Could you check a few things on this model? Use its own coordinates, in mm. A direction names the side the tool comes from. Round coordinates to 2 decimals unless told otherwise and drop trailing zeros. Loops run counter-clockwise (first coordinate to the right, second up) from the corner with the lowest first, then second, coordinate; pieces in that order, holes last. Notation, with made-up numbers: M 16,11.25 L 62,11.25 A13 cw 62,27.25 Z; hole C 72,-19 d6. An arc over 180 degrees is marked long. One line per item, written item: value. Start each with the question number.
Q1. Imagine slicing it at C-C (y = -18.95). Please give me the cut outline in (x, z).
Q2. Thinking about a two-plate mould opening in Y: for faces 1 (the face through (1.52, -22.24, 19.24)), 2 (the face through (1, -25, 28)), 3 (the face through (1, -35, 23)), which applies, released by +Y, released by -Y, zero draft, split by the parting line, or undercut?
Q3. I'm going to push flat-ended pins straight in: pin 1 Ø1.4 at (x, y) = (1, -33) entering from +Z; pin 2 Ø3 at (y, z) = (0, -21) entering from +X; pin 3 Ø1.5 at (x, z) = (1.5, 26.5) entering from +Y; pin 4 Ø0.9 at (x, y) = (1.5, -17) entering from -Z. Where does each tip first touch, or does it pass through?
Q4. Please list where these lines run through material, in increasing order: line 1 along Y through (x, z) = (0.65, -4); line 2 along Y through (x, z) = (0.4, 25.5); line 3 along Y through (x, z) = (0.95, 21).
Q5. Imagine slicing it at B-B (y = 0). Please give me the cut outline in (x, z).
Q6. Imagine slicing it at A-A (z = -21). Please give me the cut outline in (x, y).
Q7. Which directions (+Z, -Z, +X, -X, +Y, -Y) give clear straight access to the entire face, cutting with the end or side of a thin tool? Please do faces 4 (the face through (1, 10, 0)), 5 (the face through (1, -5, 27)), 6 (the face through (1.48, 2.42, -11.36)).
Q8. Imagine slicing it at D-D (x = 1.1). Give the number of separate pieces and of enclosed holes in the cut face, then the cut area to 3 significant figures.
from build123d import *

# Parameters (mm, degrees)
SKETCH_1_R      = 1.55
EXTRUDE_1_DEPTH = 3
FILLET_1_R      = 1
FILLET_2_R      = 2


with BuildPart() as part:
    # 草图1 → 凸台-拉伸1 (new body)
    with BuildSketch(Plane(origin=(0, 0, 0), x_dir=(0, 0, -1), z_dir=(1, 0, 0))):
        with BuildLine():
            Line((-8, -10), (25, -10))
            Line((25, -10), (25, 10))
            Line((25, 10), (-25, 10))
            Line((-25, 10), (-25, 7.1))
            ThreePointArc((-25, 7.1), (-23.95, 6.05), (-25, 5))
            Line((-25, 5), (-28, 5))
            Line((-28, 5), (-28, -5))
            Line((-28, -5), (-25, -5))
            ThreePointArc((-25, -5), (-23.95, -6.05), (-25, -7.1))
            Line((-25, -7.1), (-25, -17.9))
            ThreePointArc((-25, -17.9), (-23.95, -18.95), (-25, -20))
            Line((-25, -20), (-28, -20))
            Line((-28, -20), (-28, -30))
            Line((-28, -30), (-25, -30))
            ThreePointArc((-25, -30), (-23.95, -31.05), (-25, -32.1))
            Line((-25, -32.1), (-25, -35))
            Line((-25, -35), (-20, -35))
            Line((-20, -35), (-8, -14.215390309))
            Line((-8, -14.215390309), (-8, -10))
        make_face()
        with Locations((-21, 0)):
            Circle(SKETCH_1_R, mode=Mode.SUBTRACT)
        Polygon((-4.506939094, 0), (-17, -4.409315614), (-17, 4.409315614), align=None, mode=Mode.SUBTRACT)
        Polygon((12.493060906, -6), (-12.493060906, -6), (0, -1.590684386), align=None, mode=Mode.SUBTRACT)
        Polygon((0, 1.590684386), (-12.493060906, 6), (12.493060906, 6), align=None, mode=Mode.SUBTRACT)
        Polygon((17, 4.409315614), (17, -4.409315614), (4.506939094, 0), align=None, mode=Mode.SUBTRACT)
        with Locations((21, 0)):
            Circle(SKETCH_1_R, mode=Mode.SUBTRACT)
        Polygon((-20, -25), (-20, -11), (-11.917096231, -11), align=None, mode=Mode.SUBTRACT)
    extrude(amount=EXTRUDE_1_DEPTH)

    # 圆角1
    fillet_1_edges = [part.edges().sort_by_distance(p)[0] for p in [
        (1.5, -11, 20),
        (1.5, -25, 20),
        (1.5, -11, 11.917096231),
        (1.5, 6, -12.493060906),
        (1.5, 6, 12.493060906),
        (1.5, 1.590684386, 0),
        (1.5, -4.409315614, 17),
        (1.5, 0, 4.506939094),
        (1.5, 4.409315614, 17),
        (1.5, -4.409315614, -17),
        (1.5, 4.409315614, -17),
        (1.5, 0, -4.506939094),
        (1.5, -6, 12.493060906),
        (1.5, -6, -12.493060906),
        (1.5, -1.590684386, 0),
        (1.5, -10, -25),
    ]]
    fillet(fillet_1_edges, radius=FILLET_1_R)

    # 圆角2
    fillet_2_edges = [part.edges().sort_by_distance(p)[0] for p in [
        (1.5, -10, 8),
    ]]
    fillet(fillet_2_edges, radius=FILLET_2_R)


solid = part.part
Report:
1. outline: M 0,10.73 L 3,10.73 L 3,16.51 L 0,16.51 Z; M 0,20 L 3,20 L 3,23.95 L 0,23.95 Z
2. face 1: undercut
2. face 2: zero draft
2. face 3: released by -Y
3. pin 1: stops at z = 25
3. pin 2: passes through
3. pin 3: stops at y = 5
3. pin 4: stops at z = 9.35
4. line 1: y = -10 to -6, -3 to 3, 6 to 10
4. line 2: y = -30 to -20, -5 to 5
4. line 3: y = -35 to -1.55, 1.55 to 10
5. outline: M 0,-25 L 3,-25 L 3,-22.55 L 0,-22.55 Z; M 0,-19.45 L 3,-19.45 L 3,-17 L 0,-17 Z; M 0,-6.51 L 3,-6.51 L 3,6.51 L 0,6.51 Z; M 0,17 L 3,17 L 3,19.45 L 0,19.45 Z; M 0,22.55 L 3,22.55 L 3,28 L 0,28 Z
6. outline: M 0,-10 L 3,-10 L 3,-1.55 L 0,-1.55 Z; M 0,1.55 L 3,1.55 L 3,10 L 0,10 Z
7. face 4: +Z, -Z, +X, -X, +Y
7. face 5: +Z, +X, -X
7. face 6: +X, -X
8. separate pieces: 1
8. enclosed holes: 7
8. area: 1,090 mm²
